Check sheet for the drawn part. Datum: minimum x, y, z corner. Units: mm. A direction names the side the tool comes from. Coordinates: 2 decimals unless noted, no trailing zeros. Order: outer loops, then holes, each group sorted by start corner. A loop starts at its lowest first (then second) coordinate and runs counter-clockwise, first axis right, second up. Notation, with made-up numbers: M 11,79.25 L 40,79.25 A17 ccw 40,102.25 Z; hole C 71,5 d10. An arc over 180 degrees is marked long. Use one line per item in the form item = value. Start each with the question number.
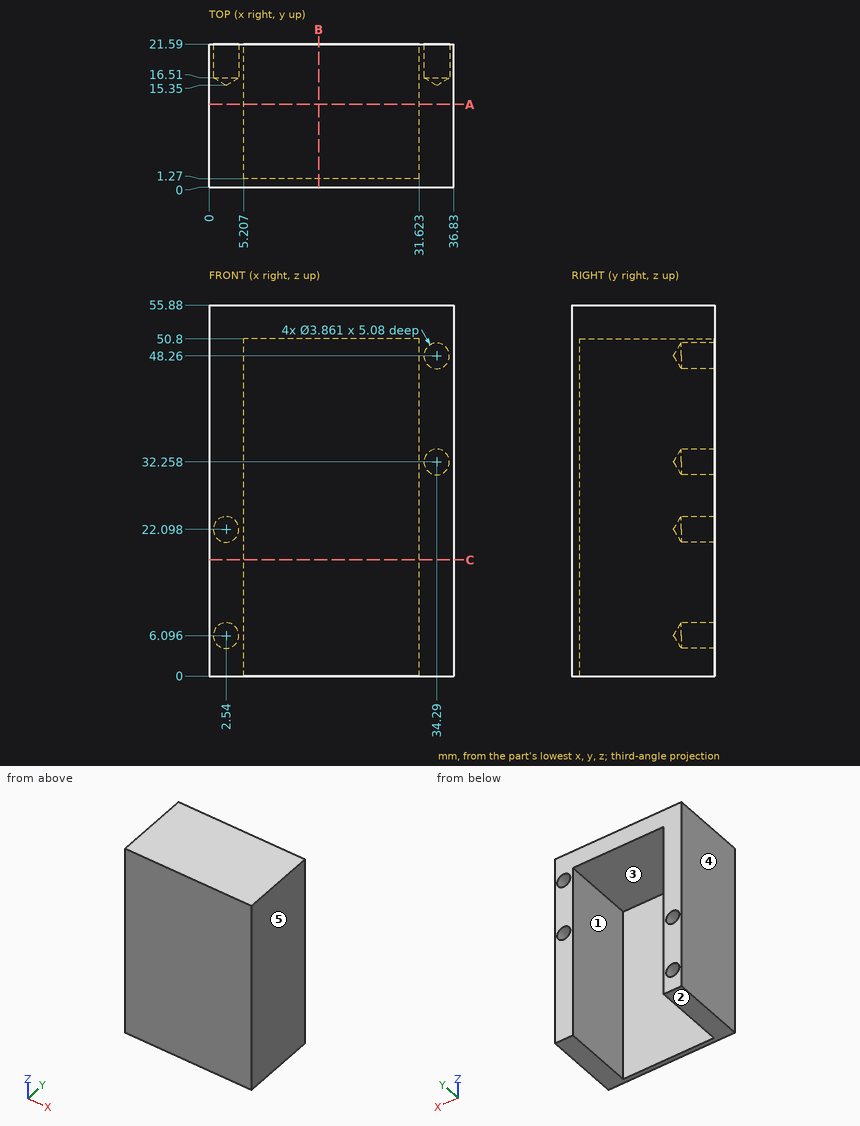
1. Cross-section at B-B on x = 16.5. Enter the section's corners in (y, z), and give its area (3 significant figures).
2. Release check for a two-part mould opening along X. For the marked faces 3, 4 and 5 record: pulls with the +X half, pulls with the -X half, needs draft (parallel to the pull), parting line crosses it, or undercut.
3. Cross-section at C-C on z = 17.5. Enter the section's corners in (x, y), and give its area (3 significant figures).
4. Material ranges on line 1 along Z through (x, y) = (2.54, 19.95); line 2 along Z through (x, y) = (34.29, 19.5); line 3 along X through (y, z) = (2.75, 6), recorded low to high.
5. Depth check by flat-ended pin: P1, Ø3, axis at x = 9, y = 7, coming from the -Z side; P2, Ø8, axis at x = 12, z = 13.5, coming from the +Y side; P3, Ø3, axis at x = 2.54, z = 6.096, coming from the +Y side. Enter the tip coordinate at first touch or a pass-through.
6. Cross-section at A-A on y = 12.5. Enter the section's corners in (x, z).
7. Tool access check on the marked faces 1 and 2. Record the directions out of +Z, -Z, +X, -X, +Y, -Y that give a thin tool (end or side, any length) a straight path to the whole face; none if there is none.
Final values:
q1.outline = M 0,0 L 1.27,0 L 1.27,50.8 L 21.59,50.8 L 21.59,55.88 L 0,55.88 Z
q1.area = 174 mm2
q2.face_3 = undercut
q2.face_4 = pulls with the -X half
q2.face_5 = pulls with the +X half
q3.outline = M 0,0 L 36.83,0 L 36.83,21.59 L 31.62,21.59 L 31.62,1.27 L 5.21,1.27 L 5.21,21.59 L 0,21.59 Z
q3.area = 258 mm2
q4.line_1 = 0 to 4.17, 8.03 to 20.17, 24.03 to 55.88
q4.line_2 = 0 to 30.33, 34.19 to 46.33, 50.19 to 55.88
q4.line_3 = 0 to 5.21, 31.62 to 36.83
q5.P1 = 50.8
q5.P2 = 1.27
q5.P3 = 16.25
q6.outline = M 0,0 L 5.21,0 L 5.21,50.8 L 31.62,50.8 L 31.62,0 L 36.83,0 L 36.83,55.88 L 0,55.88 Z
q7.face_1 = -Z, +Y
q7.face_2 = -Z, +X, -X, +Y, -Y
